Source: CAD feature listing. Evaluate the final solid. Frame: model axes, mm. Face numbers are marked on the shaded views. A direction names the side the tool comes from. Round coordinates to 2 decimals unless told otherwise and drop trailing zeros. Order: outer loops, then holes, each group sorted by start corner. A loop starts at its lowest first (then second) coordinate and runs counter-clockwise, first axis right, second up. Notation, with made-up numbers: M 12.25,1.5 L 56.25,1.5 A35 ccw 56.25,35.5 Z; hole C 27.25,-38.5 d10. An arc over 180 degrees is marked long. Answer in a Markdown table with one row per item. Add a question column.
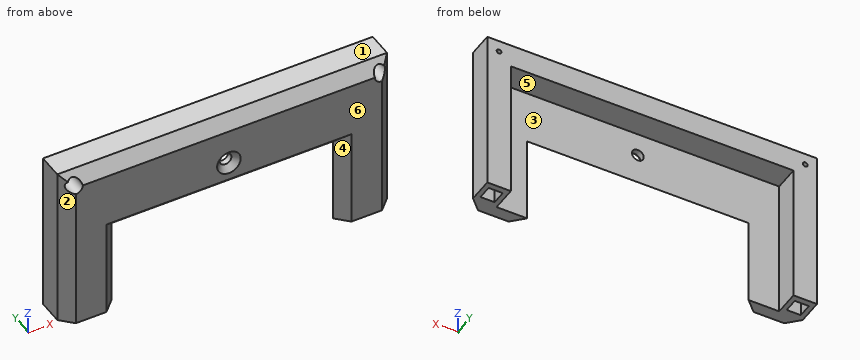
```python
from build123d import *

# Parameters (mm, degrees)
F0_W        = 140
F0_H        = 252.5
F0_R        = 1
F0_W_2      = 94
F0_H_2      = 152.5
F0_R_2      = 2.5
F0_W_3      = 12
F0_H_3      = 34
F1_DEPTH    = 15.56
F2_DEPTH    = 10.56
F3_T1_DEPTH = 165.7168298797
F3_T3_DEPTH = 278.2168298797
F4_SIZE     = 2.5
F5_R        = 3
F6_DEPTH    = 10
F7_SIZE     = 4.99999
F8_W        = 161.2529857084
F8_H        = 182.5
F9_DEPTH    = 25
F11_W       = 6
F11_H       = 50
F12_DEPTH   = 6


# Not quite as in the source:
# - a fillet or chamfer that OpenCascade refuses, or shapes differently, is made with other operations: its cross-section is extruded or revolved along the edge and cut away or added
# - a fillet or chamfer is up to 0.001 mm smaller than in the source, because OpenCascade refuses the exact size
# - a feature names something its author has since deleted; it is built from what else it names


with BuildPart() as f1:
    # F0 (on Front) → F1 (new body)
    with BuildSketch(Plane.XZ):
        with Locations((-70, 126.25)):
            Rectangle(F0_W, F0_H)
        with Locations((-135, 5)):
            Circle(F0_R, mode=Mode.SUBTRACT)
        with Locations((-5, 5)):
            Circle(F0_R, mode=Mode.SUBTRACT)
        with Locations((-135, 247.5)):
            Circle(F0_R, mode=Mode.SUBTRACT)
        Polygon((-130, 44), (-130, 242.5), (-10, 242.5), (-10, 44), (-64, 44), (-64, 10), (-76, 10), (-76, 44), align=None, mode=Mode.SUBTRACT)
        with Locations((-5, 247.5)):
            Circle(F0_R, mode=Mode.SUBTRACT)
        Polygon((-10, 242.5), (-130, 242.5), (-130, 44), (-76, 44), (-64, 44), (-10, 44), align=None)
        with Locations((-70, 143.25)):
            Rectangle(F0_W_2, F0_H_2, mode=Mode.SUBTRACT)
        with Locations((-70, 232.5)):
            Circle(F0_R_2, mode=Mode.SUBTRACT)
        with Locations((-70, 27)):
            Rectangle(F0_W_3, F0_H_3)
    extrude(amount=F1_DEPTH)

    # F0 (on Front) → F2 (cut)
    with BuildSketch(Plane.XZ):
        Polygon((-10, 242.5), (-130, 242.5), (-130, 44), (-76, 44), (-64, 44), (-10, 44), align=None)
        with Locations((-70, 143.25)):
            Rectangle(F0_W_2, F0_H_2, mode=Mode.SUBTRACT)
        with Locations((-70, 232.5)):
            Circle(F0_R_2, mode=Mode.SUBTRACT)
        with Locations((-70, 27)):
            Rectangle(F0_W_3, F0_H_3)
    extrude(amount=F2_DEPTH, mode=Mode.SUBTRACT)

    # F3: chamfer of 5 on 4 edges, made by hand

    # F3_s2 → F3_t1 (cut)
    with BuildSketch(Plane.YZ.offset(-152.8584149398)):
        Polygon((-10.56, 0), (-15.56, 5), (-15.56, 0), align=None)
        Polygon((-15.56, 247.5), (-10.56, 252.5), (-15.56, 252.5), align=None)
    extrude(amount=F3_T1_DEPTH, mode=Mode.SUBTRACT)

    # F3_s4 → F3_t3 (cut)
    with BuildSketch(Plane.XY.offset(-12.8584149398)):
        Polygon((-140, -10.56), (-135, -15.56), (-140, -15.56), align=None)
        Polygon((0, -10.56), (-5, -15.56), (0, -15.56), align=None)
    extrude(amount=F3_T3_DEPTH, mode=Mode.SUBTRACT)

    # F4
    f4_edges = [f1.edges().sort_by_distance(p)[0] for p in [
        (-72.5, -15.56, 232.5),
    ]]
    chamfer(f4_edges, length=F4_SIZE)

    # F5 (on face) → F6 (cut)
    with BuildSketch(Plane.XZ.offset(15.56)):
        with Locations((-135, 247.5)):
            Circle(F5_R)
        with Locations((-135, 5)):
            Circle(F5_R)
        with Locations((-5, 247.5)):
            Circle(F5_R)
        with Locations((-5, 5)):
            Circle(F5_R)
    extrude(amount=-F6_DEPTH, mode=Mode.SUBTRACT)

    # F7 (size 5 in the source; OpenCascade refuses exactly that, so slightly less here)
    f7_edges = [f1.edges().sort_by_distance(p)[0] for p in [
        (-70, -15.56, 67),
        (-117, -15.56, 143.25),
        (-23, -15.56, 143.25),
        (-70, -15.56, 219.5),
    ]]
    chamfer(f7_edges, length=F7_SIZE)

    # F8 (on face) → F9 (cut)
    with BuildSketch(Plane.XZ.offset(15.56)):
        with Locations((-74.815297965, 91.25)):
            Rectangle(F8_W, F8_H)
    extrude(amount=-F9_DEPTH, mode=Mode.SUBTRACT)

    # F11 (on offset) → F12 (cut)
    with BuildSketch(Plane(origin=(0, -2.5, 0), x_dir=(-1, 0, 0), z_dir=(0, 1, 0))):
        with Locations((135, 182.5)):
            Rectangle(F11_W, F11_H)
        with Locations((5, 182.5)):
            Rectangle(F11_W, F11_H)
    extrude(amount=-F12_DEPTH, mode=Mode.SUBTRACT)


solid = f1.part
```
(1) Cut plane B-B (z = 203.5). Count the separate pieces of the cut face and the enclosed holes in it, and give its area (3 significant figures).
(2) Draft query along X for the marked faces 1, 2 and 3. Return one class per face: +X half, -X half, draft (parallel to the pull), parting line (faces both ways), or undercut.
(3) Access query for the marked faces 4, 5 and 6. Directions: +Z, -Z, +X, -X, +Y, -Y. A direction counts if a zero-diameter tool reaches every point of the face in a straight line with its end or side. Return the directions, or none.
(4) Cut plane C-C (z = 232.5). Return loops of the section in (x, y), and give its area (3 significant figures).
(5) Pin query (flat end, axial travel): pin 1 (6 mm diameter, centred on y = -8, z = 199, fed in from +X); pin 2 (1.2 mm diameter, centred on x = -135, z = 247.5, fed in from +Y); pin 3 (1.5 mm diameter, centred on x = -80, z = 233.5, fed in from +Y); pin 4 (3 mm diameter, centred on x = -134, z = 247.5, fed in from -Y). Return the tip coordinate at first contact, or that it passes through.
(6) Cut plane D-D (z = 241). Return loops of the section in (x, y), and give its area (3 significant figures).
(7) Line query: line 1 (X direction, y = -3.85, z = 247.5); line 2 (X direction, y = -6, z = 226); line 3 (Z direction, x = -135, y = -7.25). Output: solid intervals per line, ascending. Write a range as from..to.
Answer list:
| question | item | result |
|---|---|---|
| 1 | separate pieces | 2 |
| 1 | enclosed holes | 2 |
| 1 | area | 319 mm² |
| 2 | face 1 | draft |
| 2 | face 2 | -X half |
| 2 | face 3 | undercut |
| 3 | face 4 | -Z, -Y |
| 3 | face 5 | -Z, +Y |
| 3 | face 6 | +Z, -Z, +X, -X, -Y |
| 4 | outline | M -140,-10.56 L -135,-15.56 L -75,-15.56 L -72.5,-13.06 L -72.5,-10.56 L -130,-10.56 L -130,0 L -140,0 Z; M -67.5,-13.06 L -65,-15.56 L -5,-15.56 L 0,-10.56 L 0,0 L -10,0 L -10,-10.56 L -67.5,-10.56 Z |
| 4 | area | 855 mm² |
| 5 | pin 1 | x = 0 |
| 5 | pin 2 | through |
| 5 | pin 3 | y = -10.56 |
| 5 | pin 4 | y = -5.56 |
| 6 | outline | M -140,-10.56 L -135,-15.56 L -5,-15.56 L 0,-10.56 L 0,0 L -10,0 L -10,-10.56 L -130,-10.56 L -130,0 L -140,0 Z |
| 6 | area | 886 mm² |
| 7 | line 1 | -140..-136, -134..-6, -4..0 |
| 7 | line 2 | -140..-130, -10..0 |
| 7 | line 3 | 207.5..244.5, 250.5..252.5 |
